Source: three-view drawing plus pictorial views. Frame: mm from the lowest corner of the part. A direction names the side the tool comes from. Coordinates: 2 decimals unless noted, no trailing zeros. Order: outer loops, then holes, each group sorted by start corner. A loop starts at its lowest first (then second) coordinate and runs counter-clockwise, first axis right, second up. Notation, with made-up numbers: M 75.25,87 L 107.25,87 A11 ccw 107.25,92 Z; hole C -0.5,65.5 d4. An arc over 180 degrees is marked long. One line per question, with ' | ' between items.
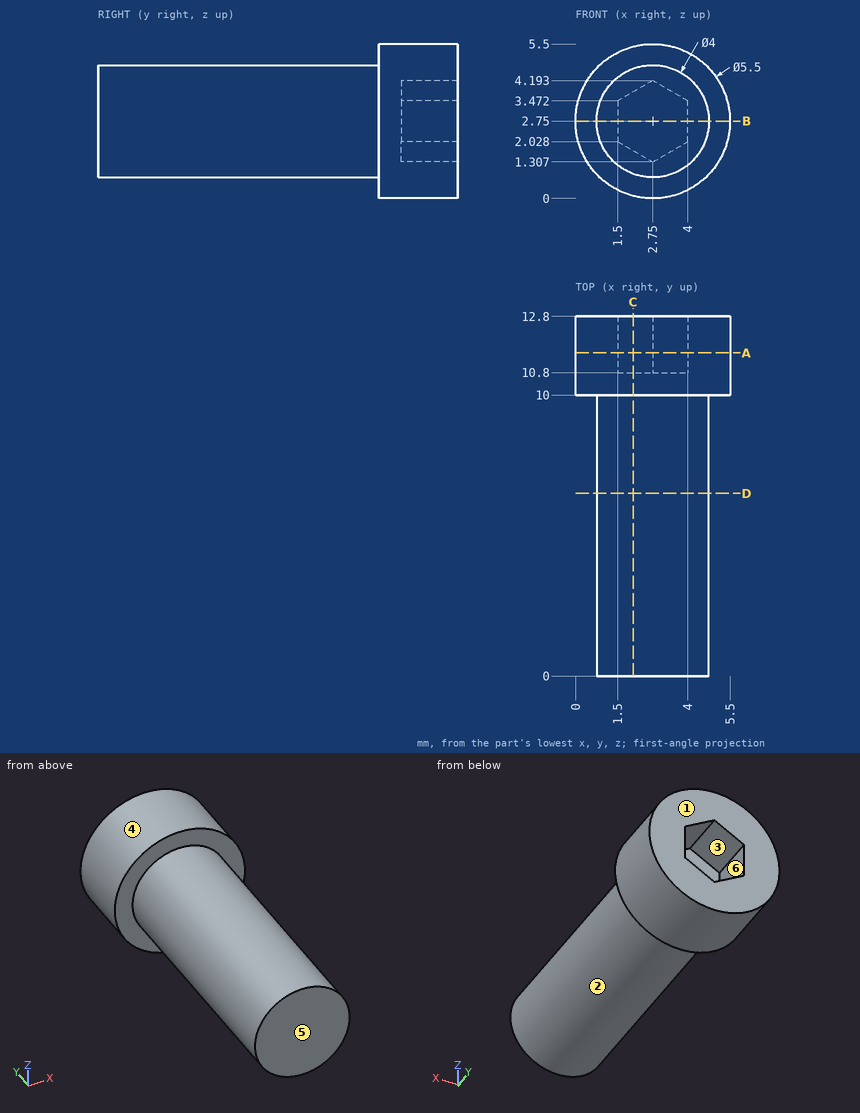
1. Access query for the marked faces 1 and 2. Directions: +Z, -Z, +X, -X, +Y, -Y. A direction counts if a zero-diameter tool reaches every point of the face in a straight line with its end or side. Return the directions, or none.
Response values:
face 1: +Z, -Z, +X, -X, +Y | face 2: -Y
2. Section B-B, the plane z = 2.75. Output: boundary loops of the cut face in (x, y), and give its area (3 significant figures).
Response values:
outline: M 0,10 L 0.75,10 L 0.75,0 L 4.75,0 L 4.75,10 L 5.5,10 L 5.5,12.8 L 4,12.8 L 4,10.8 L 1.5,10.8 L 1.5,12.8 L 0,12.8 Z | area: 50.4 mm^2
3. Section A-A, the plane y = 11.5. Output: boundary loops of the cut face in (x, z).
Response values:
outline: C 2.75,2.75 d5.5; hole M 1.5,2.03 L 2.75,1.31 L 4,2.03 L 4,3.47 L 2.75,4.19 L 1.5,3.47 Z
4. Pin query (flat end, axial travel): P1, Ø1, axis at x = 3.5, y = 5.5, coming from the -Z side; P2, Ø1, axis at x = 2, y = 10, coming from the -Z side; P3, Ø1.3, axis at x = 2.5, z = 3.5, coming from the +Y side; P4, Ø2, axis at y = 1.5, z = 3.5, coming from the -X side. Return the tip coordinate at first contact, or that it passes through.
Response values:
P1: stops at z = 0.77 | P2: stops at z = 0.01 | P3: stops at y = 12.8 | P4: stops at x = 0.75
5. Material intervals for line 1 (Y direction, x = 2.9, z = 2.15); line 2 (Y direction, x = 4.85, z = 4.3); line 3 (X direction, y = 6, z = 2.7), sorted ascending. Write a range as [from, to].
Response values:
line 1: y = [0, 10.8] | line 2: y = [10, 12.8] | line 3: x = [0.75, 4.75]
6. Draft query along Z for the marked faces 3, 4, 5 and 6. Return one class per face: pulls with the +Z half, pulls with the -Z half, needs draft (parallel to the pull), parting line crosses it, or undercut.
Response values:
face 3: undercut | face 4: parting line crosses it | face 5: needs draft | face 6: undercut
7. Section C-C, the plane x = 2.05. Output: boundary loops of the cut face in (y, z), and give its area (3 significant figures).
Response values:
outline: M 0,0.88 L 10,0.88 L 10,0.09 L 12.8,0.09 L 12.8,1.71 L 10.8,1.71 L 10.8,3.79 L 12.8,3.79 L 12.8,5.41 L 10,5.41 L 10,4.62 L 0,4.62 Z | area: 48.2 mm^2
8. Section D-D, the plane y = 6.5. Output: boundary loops of the cut face in (x, z), and give its area (3 significant figures).
Response values:
outline: C 2.75,2.75 d4 | area: 12.6 mm^2
